The listing builds one solid part. Answer for the finished solid, in the listing's coordinates (mm). A direction names the side the tool comes from. Give positions to 0.01 mm unless a question says otherwise; leave off trailing zeros. Loops run counter-clockwise (first coordinate to the right, second up) from the corner with the lowest first, then second, coordinate; pieces in that order, holes last.
Item 1: Section B-B, the plane y = 12.75 is taken. Give the vertices of the cut face in (x, z).
Item 2: Section A-A, the plane z = 24.25 is taken. Give the vertices of the cut face in (x, y), and give its area (3 significant figures).
Item 3: The mould has two halves that part along Y. Classify faces 3 (the face through (-22, 0, 13)), 4 (the face through (0, 14, 13)), 5 (the face through (-22, 14, -1.27)): pulls with the +Y half, pulls with the -Y half, needs draft (parallel to the pull), parting line crosses it, or undercut.
Item 4: Each of these flat-tipped pins is pushed along its axis until it touches: pin 1 Ø12 at (x, y) = (-17.5, 15) entering from +Z; pin 2 Ø2.5 at (x, y) = (-11.05, 16.13) entering from +Z. Where does it stop, or does it pass through?
Item 5: Section D-D, the plane x = -35 is taken. Give the vertices of the cut face in (y, z).
Item 6: Consider line 1 along X through (y, z) = (8.5, 17.5); line 2 along Y through (x, z) = (-19, 1.5); line 3 along Z through (x, y) = (-30, 8.25). Determine where each line is inside the solid, lowest interval first.
Item 7: A tool of negligible diameter and unlimited length cuts with its end or side. For faces 1 (the face through (-22, 25.4, 13)), 2 (the face through (-22, 26, 26.67)), from which of +Z, -Z, +X, -X, +Y, -Y can it reach the whole face along a straight path? Write none if from no direction.
Item 8: Section C-C, the plane x = -11.5 is taken. Give the vertices of the cut face in (y, z).
from build123d import *

# Parameters (mm, degrees)
F0_W     = 43.18
F0_H     = 2.54
F0_W_2   = 2.54
F0_H_2   = 22.86
F1_DEPTH = 26.67
F2_W     = 48.26
F2_H     = 27.94
F2_R     = 1.5875
F3_DEPTH = 1.27


with BuildPart() as f1:
    # F0 (on Top) → F1 (new body)
    with BuildSketch(Plane.XY):
        with Locations((-21.59, 26.67)):
            Rectangle(F0_W, F0_H)
        with Locations((-44.45, 26.67)):
            Rectangle(F0_W_2, F0_H)
        with Locations((-44.45, 13.97)):
            Rectangle(F0_W_2, F0_H_2)
        with Locations((-44.45, 1.27)):
            Rectangle(F0_W_2, F0_H)
        with Locations((-21.59, 1.27)):
            Rectangle(F0_W, F0_H)
        with Locations((1.27, 1.27)):
            Rectangle(F0_W_2, F0_H)
        with Locations((1.27, 13.97)):
            Rectangle(F0_W_2, F0_H_2)
        with Locations((1.27, 26.67)):
            Rectangle(F0_W_2, F0_H)
    extrude(amount=F1_DEPTH)

    # F2 (on face) → F3 (join)
    with BuildSketch(Plane(origin=(0, 0, 0), x_dir=(1, 0, 0), z_dir=(0, 0, -1))):
        with Locations((-21.59, -13.97)):
            Rectangle(F2_W, F2_H)
        with Locations((-11.054569, -16.12987)):
            Circle(F2_R, mode=Mode.SUBTRACT)
    extrude(amount=F3_DEPTH)


solid = f1.part
Worked answers:
1. outline: (-45.72, -1.27) - (2.54, -1.27) - (2.54, 26.67) - (0, 26.67) - (0, 0) - (-43.18, 0) - (-43.18, 26.67) - (-45.72, 26.67) - close
2. outline: (-45.72, 0) - (2.54, 0) - (2.54, 27.94) - (-45.72, 27.94) - close; hole (-43.18, 2.54) - (0, 2.54) - (0, 25.4) - (-43.18, 25.4) - close
2. area: 361 mm2
3. face 3: pulls with the -Y half
3. face 4: undercut
3. face 5: needs draft
4. pin 1: stops at z = 0
4. pin 2: passes through
5. outline: (0, -1.27) - (27.94, -1.27) - (27.94, 26.67) - (25.4, 26.67) - (25.4, 0) - (2.54, 0) - (2.54, 26.67) - (0, 26.67) - close
6. line 1: x = -45.72 to -43.18, 0 to 2.54
6. line 2: y = 0 to 2.54, 25.4 to 27.94
6. line 3: z = -1.27 to 0
7. face 1: +Z
7. face 2: +Z, +X, -X, +Y, -Y
8. outline: (0, -1.27) - (14.61, -1.27) - (14.61, 0) - (2.54, 0) - (2.54, 26.67) - (0, 26.67) - close; (17.65, -1.27) - (27.94, -1.27) - (27.94, 26.67) - (25.4, 26.67) - (25.4, 0) - (17.65, 0) - close
